Solid Edge part; units mm, degrees
sketch "Sketch1" plane through (0, 0, 0) normal (0, 0, 1) x (1, 0, 0)
  line L0 (-44.5263, -10.4211) -> (-44.5263, 65.3958)
  line L1 (-44.5263, 65.3958) -> (105.4737, 24.5789)
  line L2 (105.4737, 24.5789) -> (105.4737, -10.4211)
  line L3 (105.4737, -10.4211) -> (-44.5263, -10.4211)
  dimension "D1" = 105.4737
  dimension "D2" = 105.4737
extrude "Protrusion1" add sketch "Sketch1" along normal blind 75
hole "Hole_1" at (70.4737, -10.4211, 56.25) direction (0, 1, 0) diameter 6.647 depth 20
hole "Hole1" at (30.4737, -10.4211, 56.25) direction (0, 1, 0) diameter 6.647 depth 20
hole "Hole2" at (-9.5263, -10.4211, 18.75) direction (0, 1, 0) diameter 6.647 depth 20
hole "Hole3" at (30.4737, -10.4211, 18.75) direction (0, 1, 0) diameter 6.647 depth 20
hole "Hole4" at (70.4737, -10.4211, 18.75) direction (0, 1, 0) diameter 6.647 depth 20
hole "Hole5" at (-9.5263, -10.4211, 56.25) direction (0, 1, 0) diameter 6.647 depth 20
hole "Hole_14" at (3.745, 52.2606, 43.2164) direction (-0.2626, -0.9649, 0) diameter 6.647 depth 20
hole "Hole6" at (24.9579, 46.4883, 9.7994) direction (-0.2626, -0.9649, 0) diameter 6.647 depth 20
hole "Hole7" at (57.2024, 37.7142, 31.7836) direction (-0.2626, -0.9649, 0) diameter 6.647 depth 20
hole "Hole8" at (35.9895, 43.4865, 65.2006) direction (-0.2626, -0.9649, 0) diameter 6.647 depth 20
hole "Hole9" at (14.3514, 49.3744, 26.5079) direction (-0.2626, -0.9649, 0) diameter 6.647 depth 20
hole "Hole10" at (46.5959, 40.6003, 48.4921) direction (-0.2626, -0.9649, 0) diameter 6.647 depth 20
hole "Hole11" at (19.8672, 47.8735, 54.2085) direction (-0.2626, -0.9649, 0) diameter 6.647 depth 20
hole "Hole12" at (41.0801, 42.1012, 20.7915) direction (-0.2626, -0.9649, 0) diameter 6.647 depth 20
hole "Hole13" at (30.4737, 44.9874, 37.5) direction (-0.2626, -0.9649, 0) diameter 6.647 depth 20
Geometry: final body of the model. Coordinates: model frame, mm. A direction names the side the tool comes from. Round coordinates to 2 decimals unless told otherwise and drop trailing zeros. Loops run counter-clockwise (first coordinate to the right, second up) from the corner with the lowest first, then second, coordinate; pieces in that order, holes last. Notation, with made-up numbers: M 61.5,-4.5 L 68.5,-4.5 A21 cw 68.5,21.5 Z; hole C 83,60.25 d7. An arc over 180 degrees is marked long. Put each result on its own line as item: value. Start each with the question number.
(1) Section query B-B (x = -18.5). Return loops of the section in (y, z), then the cut area to 3 significant figures.
(2) Set-up query: faces 5 (the face through (19.661, 27.202, 9.753)), 6 (the face through (-10, 9.579, 19)), 7 (the face through (105.474, 7, 37)). Return all of +Z, -Z, +X, -X, +Y, -Y with unobstructed straight access to the full face (end or side cutting, diameter ignored); none if empty.
(3) Contact query for flat-ended pins moving along their axis: pin 1 Ø1 at (x, z) = (69.5, 37) entering from +Y; pin 2 Ø8.5 at (x, z) = (70.47, 18.75) entering from +Y; pin 3 Ø3.5 at (x, z) = (71.5, 56) entering from -Y. Output: stop coordinate, or through.
(4) Draft query along X for faces 1 (the face through (-44.526, 27, 37)), 2 (the face through (35.783, 22.815, 20.745)), 3 (the face through (18.43, 37.76, 57.28)), 4 (the face through (32, -10.421, 37)). Return one class per face: +X half, -X half, draft (parallel to the pull), parting line (faces both ways), or undercut.
(5) Section query A-A (y = -2.5). Return loops of the section in (x, z), then the cut area to 3 significant figures.
(6) Material intervals for line 1 along X through (y, z) = (-5.75, 18.75); line 2 along X through (y, z) = (5, 18); line 3 along Y through (x, z) = (78, 58), sorted ascending. Write a range as [from, to].
Findings below:
1. outline: M -10.42,0 L 58.31,0 L 58.31,75 L -10.42,75 Z
1. area: 5,160 mm2
2. face 5: none
2. face 6: -Y
2. face 7: +Z, -Z, +X, +Y, -Y
3. pin 1: stops at y = 34.5
3. pin 2: stops at y = 35.26
3. pin 3: stops at y = 9.58
4. face 1: -X half
4. face 2: undercut
4. face 3: undercut
4. face 4: draft
5. outline: M -44.53,0 L 105.47,0 L 105.47,75 L -44.53,75 Z; hole C -9.53,18.75 d6.65; hole C -9.53,56.25 d6.65; hole C 30.47,18.75 d6.65; hole C 30.47,56.25 d6.65; hole C 70.47,18.75 d6.65; hole C 70.47,56.25 d6.65
5. area: 11,000 mm2
6. line 1: x = [-44.53, -12.85], [-6.2, 27.15], [33.8, 67.15], [73.8, 105.47]
6. line 2: x = [-44.53, -12.76], [-6.29, 27.24], [33.71, 67.24], [73.71, 105.47]
6. line 3: y = [-10.42, 32.05]
